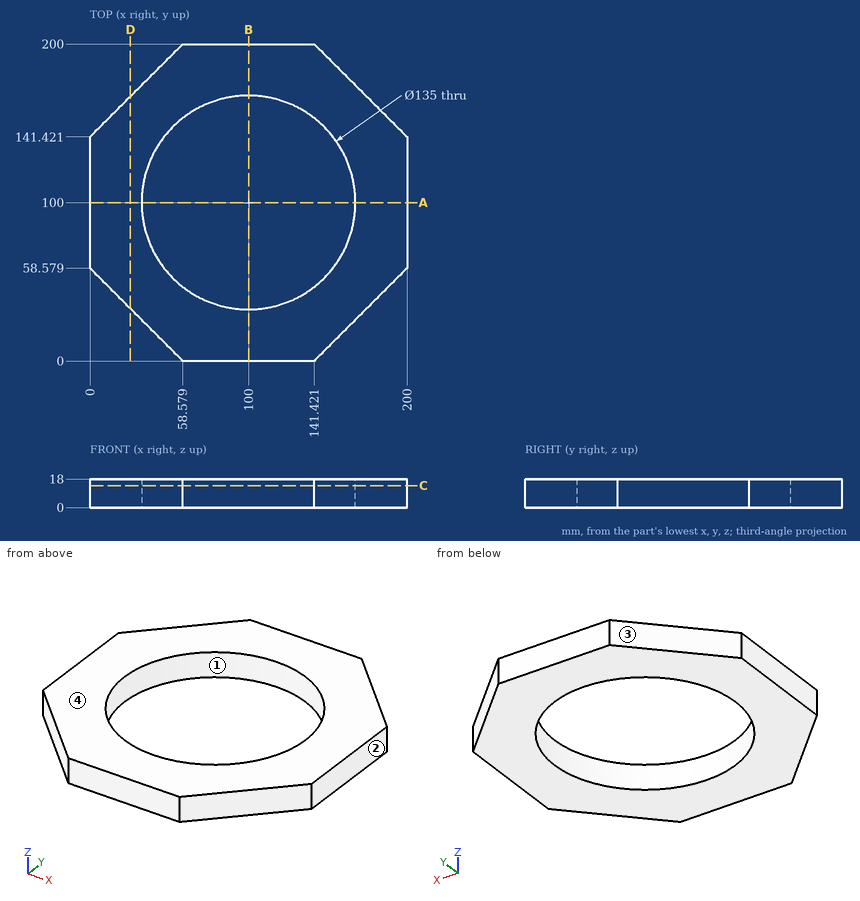
Here's the drawing with two shaded views (mm, measured from the low corner). I have some questions. Coordinates: 2 decimals unless noted, no trailing zeros. Write each loop counter-clockwise with the first axis right and the second up, starting at its lowest first coordinate (ties: lowest second). Pieces come first, ordered by that corner, then holes. Notation, with made-up numbers: (7.5, -20.75) -> (54.5, -20.75) arc R25 cw to (54.5, -1.75) -> close; hole circle Ø1 at (-18, 31). An arc over 180 degrees is marked (long way). Write item = value, one per line. Start each with the question number.
(1) I need wall thicknesses on line 1 (Y direction, x = 101, z = 11); line 2 (Y direction, x = 41, z = 4.25) (1 decimal); line 3 (X direction, y = 120, z = 4.75). Which ranges of each line are inside material? Lowest first, please. Write a range as [from, to].
(2) I want a section at D-D (x = 25.5). Please give me the cut outline in (y, z), plus the area to 3 significant figures.
(3) I want a section at A-A (y = 100). Please give me the cut outline in (x, z), plus the area to 3 significant figures.
(4) We'd pull the mould along X, two halves only. Please class the marked faces 1, 2, 3 and 4: released by +X, released by -X, zero draft, split by the parting line, or undercut.
(5) Will these pins go through, and if not, where does the flat tip stop? pin 1 (1.5 mm diameter, centred on x = 143.5, z = 4, fed in from +Y); pin 2 (8 mm diameter, centred on x = 64.5, z = 14, fed in from -Y); pin 3 (3 mm diameter, centred on y = 164.5, z = 7.5, fed in from -X).
(6) I want a section at C-C (z = 13.75). Please give me the cut outline in (x, y).
Result set:
q1.line_1 = [0, 32.51], [167.49, 200]
q1.line_2 = [17.6, 67.2], [132.8, 182.4]
q1.line_3 = [0, 35.53], [164.47, 200]
q2.outline = (33.08, 0) -> (166.92, 0) -> (166.92, 18) -> (33.08, 18) -> close
q2.area = 2,410 mm2
q3.outline = (0, 0) -> (32.5, 0) -> (32.5, 18) -> (0, 18) -> close; (167.5, 0) -> (200, 0) -> (200, 18) -> (167.5, 18) -> close
q3.area = 1,170 mm2
q4.face_1 = undercut
q4.face_2 = released by +X
q4.face_3 = released by -X
q4.face_4 = zero draft
q5.pin_1 = 198.67
q5.pin_2 = 0
q5.pin_3 = 21.58
q6.outline = (0, 58.58) -> (58.58, 0) -> (141.42, 0) -> (200, 58.58) -> (200, 141.42) -> (141.42, 200) -> (58.58, 200) -> (0, 141.42) -> close; hole circle Ø135 at (100, 100)
